Geometry check sheet. Reference: drawing and pictorial views, mm from the part's lowest x, y, z. Give positions to 0.01 mm unless a question says otherwise; leave off trailing zeros. Order: outer loops, then holes, each group sorted by start corner. A loop starts at its lowest first (then second) coordinate and runs counter-clockwise, first axis right, second up.
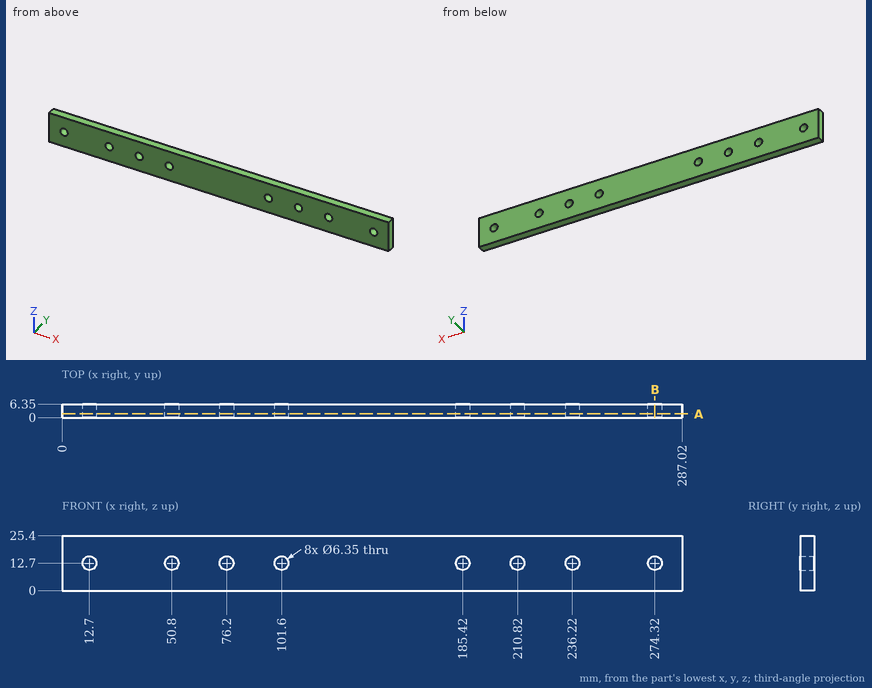
1) Section check A-A, the plane y = 1.75. State how many separate pieces and enclosed holes the cut face has, then the cut area to 3 significant figures.
Recorded:
separate pieces: 1
enclosed holes: 8
area: 7,040 mm2
2) Material ranges on L1, parallel to Z at x = 76.2, y = 4.25 (3 decimals), recorded low to high.
Recorded:
L1: z = 0 to 9.525, 15.875 to 25.4
3) Section check B-B, the plane x = 274.32. Record the cut outline in (y, z) (3 decimals), then the cut area to 3 significant figures.
Recorded:
outline: (0, 0) - (6.35, 0) - (6.35, 9.525) - (0, 9.525) - close; (0, 15.875) - (6.35, 15.875) - (6.35, 25.4) - (0, 25.4) - close
area: 121 mm2
4) Depth check by flat-ended pin: pin 1 Ø6 at (x, z) = (59.5, 19.5) entering from -Y; pin 2 Ø4 at (x, z) = (210.82, 12.7) entering from +Y. Enter the tip coordinate at first touch or a pass-through.
Recorded:
pin 1: stops at y = 0
pin 2: passes through
